Autodesk Inventor part; units mm, degrees
ref_plane "YZ Plane" through (0, 0, 0) normal (1, 0, 0) x (0, 1, 0)
ref_plane "XZ Plane" through (0, 0, 0) normal (0, 1, 0) x (-1, 0, 0)
ref_plane "XY Plane" through (0, 0, 0) normal (0, 0, 1) x (1, 0, 0)
sketch "Sketch1" plane through (0, 0, 0) normal (0, 0, 1) x (1, 0, 0)
  line L0 (-12.7, -25.4) -> (12.7, -25.4)
  line L1 (12.7, -25.4) -> (12.7, 25.4)
  line L2 (12.7, 25.4) -> (-12.7, 25.4)
  line L3 (-12.7, 25.4) -> (-12.7, -25.4)
  line L4 (-12.7, -25.4) -> (12.7, 25.4) construction
  line L5 (12.7, -25.4) -> (-12.7, 25.4) construction
  line L6 (-11.1125, 23.8125) -> (11.1125, 23.8125)
  line L7 (11.1125, 23.8125) -> (11.1125, -23.8125)
  line L8 (11.1125, -23.8125) -> (-11.1125, -23.8125)
  line L9 (-11.1125, -23.8125) -> (-11.1125, 23.8125)
  point P0 (0, 0)
  dimension "width" = 25.4
  dimension "height" = 50.8
  dimension "thickness" = 1.5875
extrude "Extrusion1" add sketch "Sketch1" along normal mid plane 152.4
sketch "Sketch2" plane through (-12.7, 25.4, 76.2) normal (0, 1, 0) x (1, 0, 0)
  line L0 (0, 152.4) -> (0, 0) construction
  line L1 (25.4, 0) -> (0, 0) construction
  line L2 (25.4, 152.4) -> (25.4, 0) construction
  line L3 (0, 152.4) -> (25.4, 152.4) construction
  line L4 (12.7, 127) -> (12.7, 25.4) construction
  point P0 (12.7, 76.2)
  point P1 (12.7, 76.2)
  point P2 (12.7, 76.2)
  dimension "d5" = 101.6
hole "Hole1" at (0, 25.4, -50.8) at (0, 25.4, 50.8) at (0, 25.4, 0) direction (0, -1, 0) diameter 5.1054 end through all
sketch "Sketch4" plane through (12.7, -25.4, 76.2) normal (1, 0, 0) x (0, 0, -1)
  circle A0 centre (76.2, 25.4) radius 53.75 construction
  line L0 (25.9391, 6.35) -> (126.4609, 6.35) construction
  line L1 (126.4609, 6.35) -> (126.4609, 44.45) construction
  line L2 (126.4609, 44.45) -> (25.9391, 44.45) construction
  line L3 (25.9391, 44.45) -> (25.9391, 6.35) construction
  line L4 (25.9391, 6.35) -> (126.4609, 44.45) construction
  line L5 (126.4609, 6.35) -> (25.9391, 44.45) construction
  line L6 (0, 0) -> (0, 50.8) construction
  dimension "d25" = 107.5
  dimension "d28" = 38.1
hole "Hole3" at (12.7, 19.05, 50.2609) at (12.7, 19.05, -50.2609) at (12.7, -19.05, -50.2609) at (12.7, -19.05, 50.2609) direction (-1, 0, 0) diameter 5.1054 end through all
sketch "Sketch5" plane through (-12.7, 25.4, 76.2) normal (0, 1, 0) x (1, 0, 0)
  line L0 (25.4, 0) -> (0, 0)
  line L1 (12.7, 136.525) -> (12.7, 15.875) construction
  line L2 (0, 152.4) -> (0, 0) construction
  point P0 (12.7, 76.2)
  point P1 (12.7, 0)
  point P2 (12.7, 76.2)
  point P3 (0, 76.2)
  dimension "d36" = 120.65
hole "Hole4" at (0, 25.4, -60.325) at (0, 25.4, 60.325) direction (0, -1, 0) diameter 5.1054 end through all
sketch "Sketch6" plane through (12.7, -25.4, 76.2) normal (1, 0, 0) x (0, 0, -1)
  circle A0 centre (126.4609, 6.35) radius 2.5527 construction
  circle A1 centre (25.9391, 44.45) radius 2.5527 construction
  circle A2 centre (126.4609, 44.45) radius 2.5527 construction
  circle A3 centre (25.9391, 6.35) radius 2.5527 construction
  line L0 (152.4, 50.8) -> (0, 50.8) construction
  line L1 (0, 0) -> (0, 50.8) construction
  line L2 (152.4, 0) -> (0, 0) construction
  line L3 (152.4, 50.8) -> (152.4, 0) construction
  circle A4 centre (126.4609, 6.35) radius 2.5527 construction
  line L4 (25.9391, 44.45) -> (126.4609, 44.45) construction
  line L5 (126.4609, 44.45) -> (126.4609, 6.35) construction
  line L6 (126.4609, 6.35) -> (25.9391, 6.35) construction
  line L7 (25.9391, 6.35) -> (25.9391, 44.45) construction
  circle A5 centre (76.2, 25.4) radius 14.2875
  dimension "d44" = 28.575
extrude "Extrusion2" cut sketch "Sketch6" against normal through all
sketch "Sketch3" plane through (12.7, -25.4, 76.2) normal (1, 0, 0) x (0, 0, -1)
  line L0 (25.9391, 44.45) -> (126.4609, 44.45) construction
  line L1 (126.4609, 44.45) -> (126.4609, 6.35) construction
  line L2 (126.4609, 6.35) -> (25.9391, 6.35) construction
  line L3 (25.9391, 6.35) -> (25.9391, 44.45) construction
  line L4 (25.9391, 44.45) -> (126.4609, 6.35) construction
  line L5 (126.4609, 44.45) -> (25.9391, 6.35) construction
  circle A0 centre (76.2, 25.4) radius 60 construction
  circle A1 centre (76.2, 25.4) radius 47.5 construction
  circle A2 centre (76.2, 25.4) radius 53.75 construction
  dimension "d16" = 107.5
  dimension "d14" = 120
  dimension "d15" = 95
  dimension "d17" = 38.1
properties part number "GP10-005" material "Aluminum 6061"
Work out the finished part from the listing and answer in its coordinate system (mm). A direction names the side the tool comes from. Coordinates: 2 decimals unless noted, no trailing zeros. Write each loop counter-clockwise with the first axis right and the second up, starting at its lowest first coordinate (ties: lowest second). Pieces come first, ordered by that corner, then holes.
Q1. A cutting plane is placed at C-C, the plane z = 50.8. State how many separate pieces and enclosed holes the cut face has, then the cut area to 3 significant figures.
Q2. A cutting plane is placed at A-A, the plane x = 7.25. Give the vertices of the cut face in (y, z).
Q3. Determine the mould class of faces 1 (the face through (-11.3, 2, 76.2)), 2 (the face through (-3, 25.4, -1)), 3 (the face through (-11.917, -17.497, -48.235)), 4 (the face through (11.9, 18.94, 52.81)) for opening direction Z: released by +Z, released by -Z, zero draft, split by the parting line, or undercut.
Q4. A cutting plane is placed at D-D, the plane y = 11.5. Give the vertices of the cut face in (x, z), then the cut area to 3 significant figures.
Q5. Find the intervals of material crossed by line 1 (Z direction, x = 12.35, y = -19.05); line 2 (Z direction, x = 0, y = -24.55); line 3 (X direction, y = 20, z = 32), in increasing order.
Q6. Which of the six approach directions +Z, -Z, +X, -X, +Y, -Y give full straight-line access (tool end or side, diameter ignored) to faces 5 (the face through (-3, 23.812, -1)), 6 (the face through (11.895, -17.497, -48.235))?
Q7. A cutting plane is placed at B-B, the plane y = -19.05. Give the vertices of the cut face in (x, z), then the cut area to 3 significant figures.
Findings below:
1. separate pieces: 6
1. enclosed holes: 0
1. area: 184 mm2
2. outline: (-25.4, -76.2) - (-23.81, -76.2) - (-23.81, 76.2) - (-25.4, 76.2) - close; (23.81, -76.2) - (25.4, -76.2) - (25.4, 76.2) - (23.81, 76.2) - close
3. face 1: released by +Z
3. face 2: zero draft
3. face 3: undercut
3. face 4: undercut
4. outline: (-12.7, -76.2) - (-11.11, -76.2) - (-11.11, -8.48) - (-12.7, -8.48) - close; (-12.7, 8.48) - (-11.11, 8.48) - (-11.11, 76.2) - (-12.7, 76.2) - close; (11.11, -76.2) - (12.7, -76.2) - (12.7, -8.48) - (11.11, -8.48) - close; (11.11, 8.48) - (12.7, 8.48) - (12.7, 76.2) - (11.11, 76.2) - close
4. area: 430 mm2
5. line 1: z = -76.2 to -52.81, -47.71 to 47.71, 52.81 to 76.2
5. line 2: z = -76.2 to -62.88, -57.77 to -53.35, -48.25 to -2.55, 2.55 to 48.25, 53.35 to 57.77, 62.88 to 76.2
5. line 3: x = -12.7 to -11.11, 11.11 to 12.7
6. face 5: +Z, -Z
6. face 6: +X, -X
7. outline: (-12.7, -76.2) - (-11.11, -76.2) - (-11.11, -52.81) - (-12.7, -52.81) - close; (-12.7, -47.71) - (-11.11, -47.71) - (-11.11, 47.71) - (-12.7, 47.71) - close; (-12.7, 52.81) - (-11.11, 52.81) - (-11.11, 76.2) - (-12.7, 76.2) - close; (11.11, -76.2) - (12.7, -76.2) - (12.7, -52.81) - (11.11, -52.81) - close; (11.11, -47.71) - (12.7, -47.71) - (12.7, 47.71) - (11.11, 47.71) - close; (11.11, 52.81) - (12.7, 52.81) - (12.7, 76.2) - (11.11, 76.2) - close
7. area: 451 mm2
